Could you check a few things on this drawing? It's one solid part, dimensions in mm from its lowest x, y, z. Round coordinates to 2 decimals unless told otherwise and drop trailing zeros. Write each loop counter-clockwise with the first axis right and the second up, starting at its lowest first coordinate (ties: lowest second). Pieces come first, ordered by that corner, then holes. Notation, with made-up numbers: (75, -29.75) - (95, -29.75) arc R21 ccw to (95, -20.75) - close; hole circle Ø3 at (53, 71.25). An arc over 180 degrees is marked (long way). Use one line per item in the form item = value. Start each with the question number.
1. We'd pull the mould along Y, two halves only. Please class the marked faces 1 and 2: +Y half, -Y half, draft (parallel to the pull), parting line (faces both ways), or undercut.
2. I want a section at A-A, the plane y = 50. List the corners of the cut face in (x, z) for me.
3. Will these pins go through, and if not, where does the flat tip stop? pin 1 (3 mm diameter, centred on y = 56.5, z = 33, fed in from +X); pin 2 (8 mm diameter, centred on x = 50, y = 79.5, fed in from +Z); pin 3 (6 mm diameter, centred on x = 68, z = 140.5, fed in from +Y).
4. I want a section at D-D, the plane z = 206.5. List the corners of the cut face in (x, y) for me, plus the area to 3 significant figures.
5. If I drill on line 1 along X through (y, z) = (50, 86); line 2 along Y through (x, z) = (52, 138); line 3 along Z through (x, y) = (48, 70.5), over which ranges is the centre line in solid material (lowest first)?
6. I want a section at C-C, the plane z = 44. List the corners of the cut face in (x, y) for me.
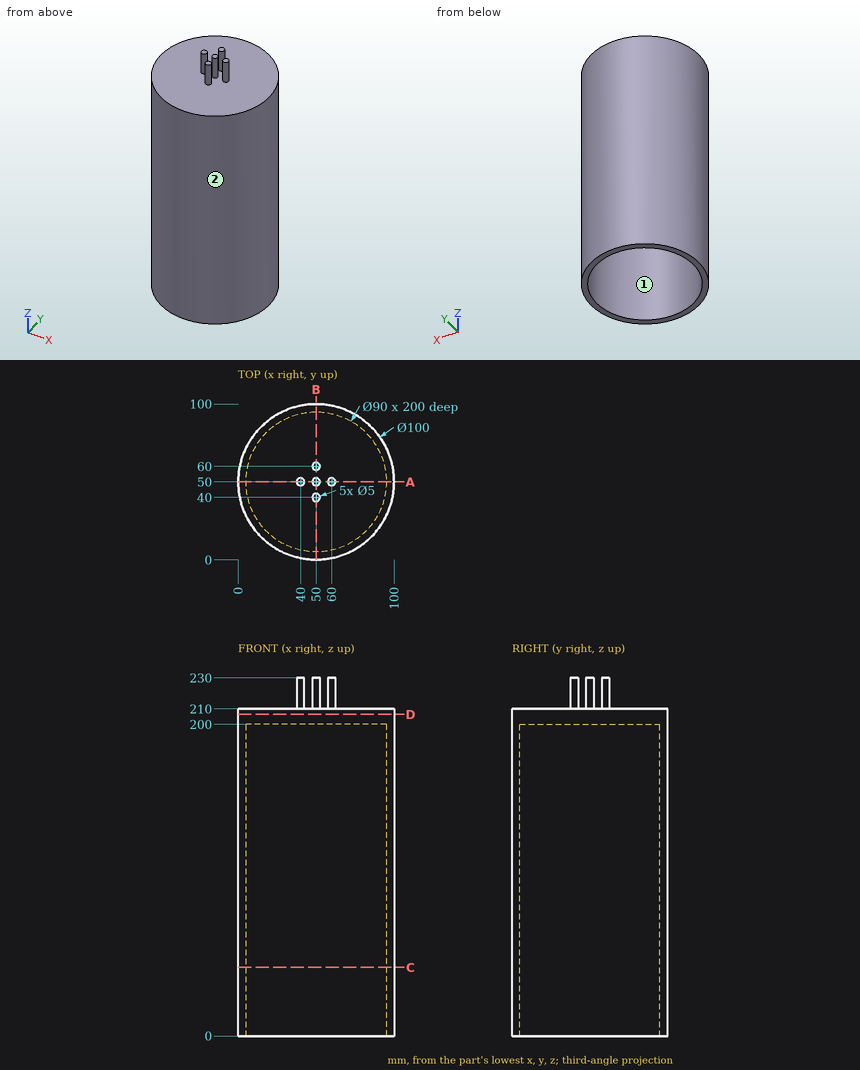
Model answer:
q1.face_1 = undercut
q1.face_2 = parting line
q2.outline = (0, 0) - (5, 0) - (5, 200) - (95, 200) - (95, 0) - (100, 0) - (100, 210) - (62.5, 210) - (62.5, 230) - (57.5, 230) - (57.5, 210) - (52.5, 210) - (52.5, 230) - (47.5, 230) - (47.5, 210) - (42.5, 210) - (42.5, 230) - (37.5, 230) - (37.5, 210) - (0, 210) - close
q3.pin_1 = 99.75
q3.pin_2 = 210
q3.pin_3 = 97.7
q4.outline = circle Ø100 at (50, 50)
q4.area = 7,850 mm2
q5.line_1 = 0 to 5, 95 to 100
q5.line_2 = 0.04 to 5.04, 94.96 to 99.96
q5.line_3 = 200 to 210
q6.outline = circle Ø100 at (50, 50); hole circle Ø90 at (50, 50)
